Read the model definition and answer for the solid it produces. Units are mm, in the model's axes. A direction names the side the tool comes from. Coordinates: 2 decimals unless noted, no trailing zeros. Write each loop counter-clockwise with the first axis right and the second up, starting at its lowest first coordinate (ties: lowest second). Pieces come first, ordered by that corner, then holes.
(1) Straight lines are drawn through the part: line 1 along Y through (x, z) = (70.5, 32); line 2 along Z through (x, y) = (-2, 25); line 3 along X through (y, z) = (-30.5, 60.5). For each, find the intervals that lie inside material, in ascending order.
(2) The part is cut by section B-B, the plane y = 0. Determine the outline of the cut face in (x, z).
(3) Determine the mould class of faces 1 (the flat face through (59, 0, 42)), 2 (the cylindrical face through (89.185, -25.21, 77.213)), 3 (the flat face through (56, -1, 60)), 4 (the flat face through (34, -11, 29)) for opening direction X: pulls with the +X half, pulls with the -X half, needs draft (parallel to the pull), parting line crosses it, or undercut.
(4) Which of the six approach directions +Z, -Z, +X, -X, +Y, -Y give full straight-line access (tool end or side, diameter ignored) to faces 5 (the flat face through (-17, 0, 30)), 6 (the flat face through (70, 10, 52)), 7 (the flat face through (34, 31, 29)), 8 (the flat face through (5, -1, 60)), 9 (the flat face through (15, 1, 53))?
(5) The part is cut by section C-C, the plane z = 53. Determine the outline of the cut face in (x, y) (3 decimals).
(6) Given pin 1 (10 mm diameter, centred on y = 1.5, z = 18, fed in from +X); pin 2 (16 mm diameter, centred on y = 20.5, z = 31.5, fed in from +X); pin 3 (8 mm diameter, centred on x = 80, y = 28.5, fed in from -Z), each flat-ended and moving along its own axis, determine where each tip first touches the part or whether it passes through.
(7) The part is cut by section D-D, the plane z = 75. Determine the outline of the cut face in (x, y), and give its area (3 significant figures).
(8) The part is cut by section A-A, the plane y = -23. Determine the outline of the cut face in (x, z).
Autodesk Fusion 360 part; units mm, degrees
sketch "Sketch1" plane through (0, 0, 0) normal (0, 0, 1) x (1, 0, 0)
  line L0 (0, 0) -> (21, 0)
  line L1 (21, 0) -> (0, 0)
  line L2 (0, 0) -> (-21, 0)
  line L3 (-21, 0) -> (-21, -40)
  line L4 (21, 0) -> (21, 40)
  line L5 (21, 40) -> (-21, 40)
  line L6 (-21, 40) -> (-21, -40)
  line L7 (-21, -40) -> (21, -40)
  line L8 (21, -40) -> (21, 40)
  dimension "d1" = 21
  dimension "d2" = 21
  dimension "d3" = 40
  dimension "d4" = 40
extrude "Extrude1" add sketch "Sketch1" along normal blind 60 makes body 1
sketch "Sketch2" plane through (0, -40, 0) normal (0, -1, 0) x (1, 0, 0)
  line L0 (-21, 0) -> (21, 0)
  line L1 (21, 0) -> (21, 60)
  line L2 (21, 60) -> (-21, 60)
  line L3 (-21, 60) -> (-21, 0)
  line L4 (-21, 60) -> (99, 60)
  line L5 (21, 0) -> (99, 60)
  dimension "d7" = 120
extrude "Extrude2" add sketch "Sketch2" against normal blind 80 contours L1 L4 L5 bodies 1
sketch "Sketch3" plane through (0, 40, 0) normal (0, 1, 0) x (-1, 0, 0)
  line L0 (-21, 0) -> (21, 0)
  line L1 (21, 0) -> (21, 60)
sketch "Sketch4" plane through (0, 0, 60) normal (0, 0, 1) x (-1, 0, 0)
  line L0 (-99, -40) -> (21, -40)
  line L1 (21, -40) -> (21, 40)
  line L2 (21, 40) -> (-99, 40)
  line L3 (-99, 40) -> (-99, -40)
  line L4 (-79, 40) -> (6, 40)
  circle A0 centre (6, 0) radius 10
  point P0 (21, 0)
  point P1 (6, 0)
  dimension "d13" = 85
  dimension "d14" = 20
extrude "Extrude3" cut sketch "Sketch4" against normal blind 234 contours A0 bodies 1
sketch "Sketch5" plane through (0, 0, 60) normal (0, 0, 1) x (-1, 0, 0)
  circle A0 centre (6, 0) radius 10
  line L0 (-99, -40) -> (21, -40)
  line L1 (21, -40) -> (21, 40)
  line L2 (21, 40) -> (-99, 40)
  line L3 (-99, 40) -> (-99, -40)
  circle A1 centre (6, 0) radius 10
  line L4 (6, -10) -> (6, 10)
  line L5 (6, -10) -> (21, -10)
  line L6 (6, 10) -> (21, 10)
extrude "Extrude4" cut sketch "Sketch5" against normal blind 30 contours A0 L1 A1 L5 L6 bodies 1
sketch "Sketch6" plane through (0, 0, 60) normal (0, 0, 1) x (-1, 0, 0)
  line L0 (21, -10) -> (6, -10)
  arc A0 (6, 10) -> (6, -10) centre (6, 0) ccw
  line L1 (6, 10) -> (21, 10)
  line L2 (21, 10) -> (21, 40)
  line L3 (21, 40) -> (-99, 40)
  line L4 (-99, 40) -> (-99, -40)
  line L5 (-99, -40) -> (21, -40)
  line L6 (21, -40) -> (21, -10)
  line L7 (21, 40) -> (-79, 40)
  line L8 (-79, 40) -> (-34, 40)
  line L9 (-99, 0) -> (-99, 21)
  line L10 (-99, 0) -> (-99, -21)
  line L11 (-24, -31) -> (-44, -31)
  line L12 (-44, -31) -> (-44, -11)
  line L13 (-44, -11) -> (-24, -11)
  line L14 (-24, -11) -> (-24, -31)
  line L15 (-24, -31) -> (-44, -11) construction
  line L16 (-44, -31) -> (-24, -11) construction
  line L17 (-44, 11) -> (-24, 11)
  line L18 (-24, 11) -> (-24, 31)
  line L19 (-24, 31) -> (-44, 31)
  line L20 (-44, 31) -> (-44, 11)
  line L21 (-44, 11) -> (-24, 31) construction
  line L22 (-24, 11) -> (-44, 31) construction
  point P0 (-99, 0)
  point P1 (-34, 21)
  point P2 (-34, -21)
  point P3 (-34, -21)
  point P4 (-34, 21)
  dimension "d23" = 20
  dimension "d24" = 20
  dimension "d25" = 20
  dimension "d26" = 20
sketch "Sketch9" plane through (0, 0, 60) normal (0, 0, 1) x (-1, 0, 0)
  line L0 (21, -10) -> (6, -10)
  arc A0 (6, 10) -> (6, -10) centre (6, 0) ccw
  line L1 (6, 10) -> (21, 10)
  line L2 (21, 10) -> (21, 40)
  line L3 (21, 40) -> (-99, 40)
  line L4 (-99, 40) -> (-99, -40)
  line L5 (-99, -40) -> (21, -40)
  line L6 (21, -40) -> (21, -10)
  line L7 (-99, 40) -> (-135, 40)
  line L8 (-135, 40) -> (-135, -40)
  line L9 (-135, -40) -> (-99, -40)
  line L10 (-99, -40) -> (-99, 40)
extrude "Extrude7" add sketch "Sketch9" against normal blind 60 separate body contours L4 L7 L8 L9 L10 makes body 2
extrude "Extrude8" add 1 faces at (99, -13.3333, 40) along direction (-1, 0, 0) blind 85 on bodies 2 bodies 2 1
extrude "Extrude5" cut sketch "Sketch6" against normal blind 75 contours L11 L12 L13 L14 | L17 L18 L19 L20 bodies 2
sketch "Sketch7" plane through (0, 0, 60) normal (0, 0, 1) x (-1, 0, 0)
  line L0 (-44, -31) -> (-44, -11)
  line L1 (-44, -11) -> (-24, -11)
  line L2 (-24, -11) -> (-24, -31)
  line L3 (-24, -31) -> (-44, -31)
  line L4 (-24, 11) -> (-44, 11)
  line L5 (-44, 11) -> (-44, 31)
  line L6 (-44, 31) -> (-24, 31)
  line L7 (-24, 31) -> (-24, 11)
  line L8 (21, -10) -> (6, -10)
  arc A0 (6, 10) -> (6, -10) centre (6, 0) ccw
  line L9 (6, 10) -> (21, 10)
  line L10 (21, 10) -> (21, 40)
  line L11 (21, 40) -> (-135, 40)
  line L12 (-135, -40) -> (21, -40)
  line L13 (21, -40) -> (21, -10)
  line L14 (-79, 40) -> (-34, 40)
  line L15 (-34, 40) -> (-53, 40)
  line L16 (-34, 40) -> (-15, 40)
  line L17 (-15, 40) -> (-53, 40)
  line L18 (-53, 40) -> (-53, -40)
  line L19 (-53, -40) -> (-15, -40)
  line L20 (-15, -40) -> (-15, 40)
  line L21 (-135, 40) -> (-135, -40)
  dimension "d30" = 45
extrude "Extrude6" cut sketch "Sketch7" against normal blind 15 contours L11 L12 L14 L15 L16 L17 L18 L19 L20 bodies 2
sketch "Sketch10" plane through (0, -40, 0) normal (0, -1, 0) x (1, 0, 0)
  line L0 (15, 45) -> (15, 60)
  line L1 (15, 60) -> (-21, 60)
  line L2 (-21, 60) -> (-21, 0)
  line L3 (-21, 0) -> (135, 0)
  line L4 (135, 0) -> (135, 60)
  line L5 (135, 60) -> (53, 60)
  line L6 (53, 60) -> (53, 45)
  line L7 (53, 45) -> (15, 45)
  circle A0 centre (79, 60) radius 20
  line L8 (-21, 0) -> (21, 0)
  line L9 (21, 0) -> (89.6293, 43.0584)
  dimension "d40" = 40
  dimension "d41" = 42
extrude "Extrude9" cut sketch "Sketch10" against normal blind 165 contours L3 L4 L5 A0 L9 bodies 2
sketch "Sketch11" plane through (0, -40, 0) normal (0, -1, 0) x (1, 0, 0)
  line L0 (21, 0) -> (89.6293, 43.0584)
  arc A0 (89.6293, 43.0584) -> (99, 60) centre (79, 60) ccw
  line L1 (99, 60) -> (53, 60)
  line L2 (53, 60) -> (53, 45)
  line L3 (53, 45) -> (15, 45)
  line L4 (15, 45) -> (15, 60)
  line L5 (15, 60) -> (-21, 60)
  line L6 (-21, 60) -> (-21, 0)
  line L7 (-21, 0) -> (21, 0)
  circle A1 centre (79, 60) radius 20
  dimension "d45" = 40
extrude "Extrude10" add sketch "Sketch11" against normal blind 80 contours A0 L1 A1 | L1 A1 bodies 2
sketch "Sketch12" plane through (0, -40, 0) normal (0, -1, 0) x (1, 0, 0)
  line L0 (59, 60) -> (53, 60)
  line L1 (53, 60) -> (53, 45)
  line L2 (53, 45) -> (15, 45)
  line L3 (15, 45) -> (15, 60)
  line L4 (15, 60) -> (-21, 60)
  line L5 (-21, 60) -> (-21, 0)
  line L6 (-21, 0) -> (21, 0)
  line L7 (21, 0) -> (89.6293, 43.0584)
  arc A0 (89.6293, 43.0584) -> (59, 60) centre (79, 60) ccw
  circle A1 centre (79, 60) radius 10
  dimension "d48" = 20
extrude "Extrude11" cut sketch "Sketch12" against normal blind 180 contours A1 bodies 2
sketch "Sketch13" plane through (0, 0, 60) normal (0, 0, 1) x (-1, 0, 0)
  line L0 (-15, 40) -> (-15, -40)
  line L1 (-15, -40) -> (21, -40)
  line L2 (21, -40) -> (21, -10)
  line L3 (21, -10) -> (6, -10)
  arc A0 (6, 10) -> (6, -10) centre (6, 0) ccw
  line L4 (6, 10) -> (21, 10)
  line L5 (21, 10) -> (21, 40)
  line L6 (21, 40) -> (-15, 40)
  line L7 (-59, 0) -> (-59, -10)
  line L8 (-59, 0) -> (-59, 10)
  line L9 (-59, -10) -> (-105, -10)
  line L10 (-105, -10) -> (-105, 10)
  line L11 (-105, 10) -> (-59, 10)
  line L12 (-59, 10) -> (-59, -10)
  dimension "d52" = 10
  dimension "d53" = 10
extrude "Extrude12" cut sketch "Sketch13" along normal blind 50 and the other way blind 60 contours L7 L8 L9 L10 L11 L12 bodies 2
Computed:
1. line 1: y = -40 to -10, 10 to 40
1. line 2: z = 0 to 60
1. line 3: x = 59.01 to 69.01, 88.99 to 98.99
2. outline: (-21, 0) - (-16, 0) - (-16, 30) - (-21, 30) - close; (4, 0) - (21, 0) - (59, 23.84) - (59, 60) - (53, 60) - (53, 45) - (15, 45) - (15, 60) - (4, 60) - close
3. face 1: pulls with the +X half
3. face 2: parting line crosses it
3. face 3: needs draft
3. face 4: undercut
4. face 5: +Z, -X
4. face 6: +Z, -Z, +X
4. face 7: +Z, -Z
4. face 8: +Z, -X, +Y, -Y
4. face 9: +Z, +Y, -Y
5. outline: (-21, -40) - (15, -40) - (15, 40) - (-21, 40) - (-21, 10) - (-6, 10) arc R10 cw to (-6, -10) - (-21, -10) - close; (53, -40) - (71.859, -40) - (71.859, -10) - (59, -10) - (59, 10) - (71.859, 10) - (71.859, 40) - (53, 40) - close; (86.141, -40) - (97.735, -40) - (97.735, -10) - (86.141, -10) - close; (86.141, 10) - (97.735, 10) - (97.735, 40) - (86.141, 40) - close
6. pin 1: stops at x = 57.66
6. pin 2: stops at x = 83.96
6. pin 3: stops at z = 34.51
7. outline: (65.77, -40) - (92.23, -40) - (92.23, -10) - (65.77, -10) - close; (65.77, 10) - (92.23, 10) - (92.23, 40) - (65.77, 40) - close
7. area: 1,590 mm2
8. outline: (-21, 0) - (21, 0) - (24, 1.88) - (24, 45) - (15, 45) - (15, 60) - (-21, 60) - close; (44, 14.43) - (89.63, 43.06) arc R20 ccw (long way) to (59, 60) - (53, 60) - (53, 45) - (44, 45) - close; hole circle Ø20 at (79, 60)
